```python
from build123d import *

# Parameters (mm, degrees)
SKETCH1_R               = 13.7
BOSS_EXTRUDE1_DEPTH     = 38
SKETCH2_R               = 18.5
BOSS_EXTRUDE2_DEPTH     = 25
SKETCH3_R               = 6
BOSS_EXTRUDE3_DEPTH     = 6.8
SKETCH4_R               = 3
BOSS_EXTRUDE4_DEPTH     = 30
SKETCH5_R               = 1.5
CUT_EXTRUDE1_DEPTH      = 0.5
CUT_EXTRUDE2_DEPTH      = 104.172380025
CUT_EXTRUDE2_DEPTH_BACK = 104.172380025
SKETCH6_R               = 1


with BuildPart() as part:
    # Sketch1 → Boss-Extrude1 (new body)
    with BuildSketch(Plane.XY):
        Circle(SKETCH1_R)
    extrude(amount=BOSS_EXTRUDE1_DEPTH)

    # Sketch2 → Boss-Extrude2 (add)
    with BuildSketch(Plane.XY.offset(38)):
        Circle(SKETCH2_R)
    extrude(amount=BOSS_EXTRUDE2_DEPTH)

    # Sketch3 → Boss-Extrude3 (add)
    with BuildSketch(Plane.XY.offset(63)):
        with Locations((0, 7)):
            Circle(SKETCH3_R)
    extrude(amount=BOSS_EXTRUDE3_DEPTH)

    # Sketch4 → Boss-Extrude4 (add)
    with BuildSketch(Plane.XY.offset(69.8)):
        with Locations((0, 7)):
            Circle(SKETCH4_R)
    extrude(amount=BOSS_EXTRUDE4_DEPTH)

    # Sketch5 → Cut-Extrude1 (cut)
    with BuildSketch(Plane.XY.offset(63)):
        with Locations((-15.75, 0)):
            Circle(SKETCH5_R)
        with Locations((-7.875, 13.63990011)):
            Circle(SKETCH5_R)
        with Locations((7.875, 13.63990011)):
            Circle(SKETCH5_R)
        with Locations((15.75, 0)):
            Circle(SKETCH5_R)
        with Locations((7.875, -13.63990011)):
            Circle(SKETCH5_R)
        with Locations((-7.875, -13.63990011)):
            Circle(SKETCH5_R)
    extrude(amount=-CUT_EXTRUDE1_DEPTH, mode=Mode.SUBTRACT)

    # Sketch6 → Cut-Extrude2 (cut, two sides: drawn at the far end of the back side and taken through both)
    with BuildSketch(Plane(origin=(0, 0, 0), x_dir=(0, 0, -1), z_dir=(1, 0, 0)).offset(-CUT_EXTRUDE2_DEPTH_BACK)):
        with Locations(Location((-91.8, 7, 0), (0, 0, 180))):
            Circle(SKETCH6_R)
    extrude(amount=CUT_EXTRUDE2_DEPTH + CUT_EXTRUDE2_DEPTH_BACK, mode=Mode.SUBTRACT)


solid = part.part
```
Model file for the job. Use its own axes, mm. A direction names the side the tool comes from. Give positions to 0.01 mm unless a question says otherwise; leave off trailing zeros. Order: outer loops, then holes, each group sorted by start corner. A loop starts at its lowest first (then second) coordinate and runs counter-clockwise, first axis right, second up.
1) Mould opens along X. For faces 1 (the flat face through (-14, 0, 38)), 2 (the flat face through (8, -14, 62.5)), 3 (the cylindrical face through (-0.78, 12.95, 66.35)) say: +X half, -X half, draft (parallel to the pull), parting line (faces both ways), or undercut.
2) Saw through at C-C, the plane y = 0. Write the cut outline in (x, z), then the cut area to 3 significant figures.
3) 3-axis set-ups, long thin cutter, end or side, ignore diameter. For faces 4 (the cylindrical face through (-10.097, 9.259, 18.734)), 5 (the cylindrical face through (-4.01, -18.06, 50.32)), 6 (the cylindrical face through (-9.374, 13.706, 62.754)): which of +Z, -Z, +X, -X, +Y, -Y reach the whole face in a straight line?
4) Saw through at B-B, the plane y = 7. Write the cut outline in (x, z), then the cut area to 3 significant figures.
5) Saw through at A-A, the plane x = 0. Write the cut outline in (y, z).
6) Pin check, flat tips, straight feed: pin 1 (4 mm diameter, centred on x = 15.75, y = 0, fed in from +Z); pin 2 (0.9 mm diameter, centred on x = 7.5, y = 13.5, fed in from +Z); pin 3 (10 mm diameter, centred on y = 6, z = 62, fed in from -X). Stop position of each tip, or through.
7) Wall check: probe 1 along Y at (x, z) = (0, 41); probe 2 along Z at (x, y) = (-10, 7); probe 3 along Z at (x, y) = (15.5, -8). Give the ranges that are in metal, low to high.
8) Saw through at D-D, the plane z = 35. Write the cut outline in (x, y), then the cut area to 3 significant figures.
Computed:
1. face 1: draft
1. face 2: undercut
1. face 3: parting line
2. outline: (-18.5, 38) - (-13.7, 38) - (-13.7, 0) - (13.7, 0) - (13.7, 38) - (18.5, 38) - (18.5, 63) - (17.25, 63) - (17.25, 62.5) - (14.25, 62.5) - (14.25, 63) - (-14.25, 63) - (-14.25, 62.5) - (-17.25, 62.5) - (-17.25, 63) - (-18.5, 63) - close
2. area: 1,960 mm2
3. face 4: -Z
3. face 5: +Z, -Z
3. face 6: +Z
4. outline: (-17.12, 38) - (-11.78, 38) - (-11.78, 0) - (11.78, 0) - (11.78, 38) - (17.12, 38) - (17.12, 63) - (6, 63) - (6, 69.8) - (3, 69.8) - (3, 90.8) - (-3, 90.8) - (-3, 69.8) - (-6, 69.8) - (-6, 63) - (-17.12, 63) - close; (-3, 92.8) - (3, 92.8) - (3, 99.8) - (-3, 99.8) - close
4. area: 2,000 mm2
5. outline: (-18.5, 38) - (-13.7, 38) - (-13.7, 0) - (13.7, 0) - (13.7, 38) - (18.5, 38) - (18.5, 63) - (13, 63) - (13, 69.8) - (10, 69.8) - (10, 99.8) - (4, 99.8) - (4, 69.8) - (1, 69.8) - (1, 63) - (-18.5, 63) - close; hole circle Ø2 at (7, 91.8)
6. pin 1: stops at z = 63
6. pin 2: stops at z = 62.5
6. pin 3: stops at x = -18.47
7. probe 1: y = -18.5 to 18.5
7. probe 2: z = 0 to 63
7. probe 3: z = 38 to 63
8. outline: circle Ø27.4 at (0, 0)
8. area: 590 mm2
